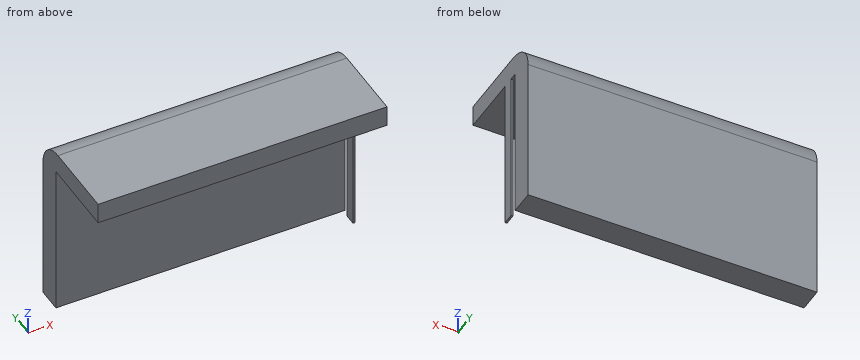
from build123d import *

# Parameters (mm, degrees)
SKETCH2_W           = 204.3
SKETCH2_H           = 73.9
BOSS_EXTRUDE1_DEPTH = 126
SKETCH3_W           = 111
SKETCH3_H           = 56.6
CUT_EXTRUDE2_DEPTH  = 274.3
FILLET1_R           = 20
SKETCH5_W           = 111
SKETCH5_H           = 7.907805674
BOSS_EXTRUDE4_DEPTH = 1.3


with BuildPart() as part:
    # Sketch2 → Boss-Extrude1 (new body)
    with BuildSketch(Plane.XY):
        with Locations((40.038337802, -14.066756032)):
            Rectangle(SKETCH2_W, SKETCH2_H)
    extrude(amount=BOSS_EXTRUDE1_DEPTH)

    # Sketch3 → Cut-Extrude2 (cut)
    with BuildSketch(Plane(origin=(142.188337802, 0, 0), x_dir=(0, 0, -1), z_dir=(1, 0, 0))):
        with Locations((-55.5, -22.716756032)):
            Rectangle(SKETCH3_W, SKETCH3_H)
    extrude(amount=-CUT_EXTRUDE2_DEPTH, mode=Mode.SUBTRACT)

    # Fillet1
    fillet1_edges = [part.edges().sort_by_distance(p)[0] for p in [
        (40.038337802, 22.883243968, 126),
    ]]
    fillet(fillet1_edges, radius=FILLET1_R)

    # Sketch5 → Boss-Extrude4 (add)
    with BuildSketch(Plane(origin=(142.188337802, 0, 0), x_dir=(0, 0, -1), z_dir=(1, 0, 0))):
        with Locations((-55.5, -3.953902837)):
            Rectangle(SKETCH5_W, SKETCH5_H)
    extrude(amount=-BOSS_EXTRUDE4_DEPTH)


solid = part.part
For this review, take the finished solid that the model builds, in its own axes (mm). Round coordinates to 2 decimals unless told otherwise and drop trailing zeros. Write each loop counter-clockwise with the first axis right and the second up, starting at its lowest first coordinate (ties: lowest second). Pieces come first, ordered by that corner, then holes. Notation, with made-up numbers: (-21, -26.75) - (11, -26.75) arc R31 ccw to (11, -1.75) - close; hole circle Ø9 at (58.5, 73.25). An arc over 180 degrees is marked (long way). Write item = value, one per line. Start each with the question number.
1. Consider section D-D on y = 12. State the section outline as (x, z) points, plus the area to 3 significant figures.
2. Wall thickness on L1, parallel to Y at x = -18, z = 92.5; L2, parallel to Z at x = -46, y = -44; L3, parallel to X at y = -4, z = 90.5: over which ranges is each line inside the solid? List them lowest first.
3. Consider section C-C on y = -42. State the section outline as (x, z) points, plus the area to 3 significant figures.
4. For pin 1 Ø6 at (x, y) = (-35.5, -14) entering from -Z; pin 2 Ø8 at (x, z) = (38.5, 81.5) entering from -Y; pin 3 Ø4 at (y, z) = (-2.5, 29.5) entering from -X, all flat-tipped, find the tip position at first contact; note any pin that passes through.
5. Consider section A-A on z = 85.5. State the section outline as (x, y) points, plus the area to 3 significant figures.
6. Consider section B-B on x = 90.5. State the section outline as (y, z) points, plus the area to 3 significant figures.
Evaluation:
q1.outline = (-62.11, 0) - (142.19, 0) - (142.19, 123.8) - (-62.11, 123.8) - close
q1.area = 25,300 mm2
q2.L1 = 5.58 to 22.88
q2.L2 = 111 to 126
q2.L3 = 140.89 to 142.19
q3.outline = (-62.11, 111) - (142.19, 111) - (142.19, 126) - (-62.11, 126) - close
q3.area = 3,060 mm2
q4.pin_1 = 111
q4.pin_2 = 5.58
q4.pin_3 = 140.89
q5.outline = (-62.11, 5.58) - (142.19, 5.58) - (142.19, 22.88) - (-62.11, 22.88) - close; (140.89, -7.91) - (142.19, -7.91) - (142.19, 0) - (140.89, 0) - close
q5.area = 3,540 mm2
q6.outline = (-51.02, 111) - (5.58, 111) - (5.58, 0) - (22.88, 0) - (22.88, 106) arc R20 ccw to (2.88, 126) - (-51.02, 126) - close
q6.area = 2,940 mm2
